Can you work these out from the model? Positions are in its coordinate system, mm. Face numbers are marked on the shaded views. A direction names the side the tool comes from. Give positions to 0.01 mm unless a question says otherwise; leave off trailing zeros. Order: outer loops, then holes, each group sorted by start corner. A loop starts at its lowest first (then second) coordinate and runs counter-clockwise, first axis right, second up. Notation, with made-up numbers: (-12, -39) - (1, -39) arc R25 ccw to (1, -5) - close; hole circle Ø5 at (-35, -29.75). An arc over 180 degrees is marked (long way). Use one line per item in the form item = value. Start each with the question number.
1) Please list where these lines run through material, in increasing order: probe 1 along Y at (x, z) = (39, 14); probe 2 along X at (y, z) = (-47, 35); probe 3 along Z at (x, y) = (90, -22).
2) Suppose I cut it at D-D, the plane y = -9.5. Write out the boundary of the cut face in (x, z), and give its area (3 significant figures).
3) Suppose I cut it at B-B, the plane y = -27. Write out the boundary of the cut face in (x, z), and give its area (3 significant figures).
4) Suppose I cut it at A-A, the plane y = -20. Write out the boundary of the cut face in (x, z), and give its area (3 significant figures).
5) Suppose I cut it at C-C, the plane x = 90. Write out the boundary of the cut face in (y, z).
6) Which directions (+Z, -Z, +X, -X, +Y, -Y) give clear straight access to the entire face, cutting with the end or side of a thin tool? Please do the marked faces 5, 6 and 7.
7) We'd pull the mould along X, two halves only. Please class the marked faces 1, 2, 3 and 4: released by +X, released by -X, zero draft, split by the parting line, or undercut.
8) For pin 1 (10 mm diameter, centred on y = -8, z = 35, fed in from -X); pin 2 (10 mm diameter, centred on x = 59, z = 23.5, fed in from +Y); pin 3 (4 mm diameter, centred on y = -21, z = 47.5, fed in from -X), each with a flat end and sliding along its axis, tell me the tip position at first contact or that it passes through.
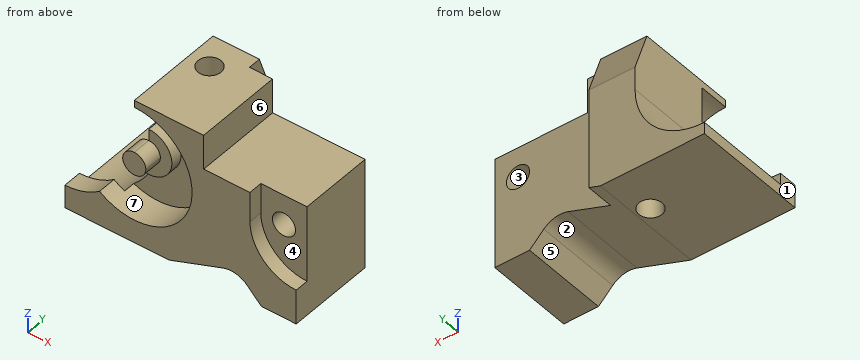
```python
from build123d import *

# Parameters (mm, degrees)
F0_W      = 100
F0_H      = 63
F1_DEPTH  = 50
F2_W      = 40
F2_H      = 15
F3_DEPTH  = 50.001
F5_DEPTH  = 6
F6_R      = 5
F7_DEPTH  = 44.001
F8_R      = 25
F9_DEPTH  = 13
F10_R     = 10
F11_DEPTH = 5
F13_DEPTH = 42
F15_DEPTH = 50.001
F17_DEPTH = 8
F19_DEPTH = 63.001
F20_R     = 5
F21_DEPTH = 63.001
F23_DEPTH = 70.001


with BuildPart() as f1:
    # F0 (on Front) → F1 (new body)
    with BuildSketch(Plane.XZ):
        with Locations((50, 31.5)):
            Rectangle(F0_W, F0_H)
    extrude(amount=F1_DEPTH)

    # F2 (on face) → F3 (cut, through all)
    with BuildSketch(Plane.XZ.offset(50)):
        with Locations((80, 55.5)):
            Rectangle(F2_W, F2_H)
        with BuildLine():
            Line((45, 0), (85, 0))
            Line((85, 0), (78.8309201782, 6.1690798218))
            ThreePointArc((78.8309201782, 6.1690798218), (73.9242485057, 8.8609720811), (68.3396509331, 8.4949382178))
            Line((68.3396509331, 8.4949382178), (45, 0))
        make_face()
    extrude(amount=-F3_DEPTH, mode=Mode.SUBTRACT)

    # F4 (on face) → F5 (cut)
    with BuildSketch(Plane.XZ.offset(50)):
        with BuildLine():
            Line((100, 48), (84.8013158464, 48))
            ThreePointArc((84.8013158464, 48), (81.2386876382, 41.9291527956), (80, 35))
            Line((80, 35), (100, 35))
            Line((100, 35), (100, 48))
        make_face()
        with BuildLine():
            ThreePointArc((80, 35), (81.2386876382, 41.9291527956), (84.8013158464, 48))
            Line((84.8013158464, 48), (80, 48))
            Line((80, 48), (80, 35))
        make_face()
        with BuildLine():
            ThreePointArc((80, 35), (85.8578643763, 20.8578643763), (100, 15))
            Line((100, 15), (100, 35))
            Line((100, 35), (80, 35))
        make_face()
    extrude(amount=-F5_DEPTH, mode=Mode.SUBTRACT)

    # F6 (on face) → F7 (cut, through all)
    with BuildSketch(Plane.XZ.offset(44)):
        with Locations((90, 35)):
            Circle(F6_R)
    extrude(amount=-F7_DEPTH, mode=Mode.SUBTRACT)

    # F8 (on face) → F9 (cut)
    with BuildSketch(Plane.XZ.offset(50)):
        with Locations((30, 35)):
            Circle(F8_R)
    extrude(amount=-F9_DEPTH, mode=Mode.SUBTRACT)

    # F10 (on face) → F11 (join)
    with BuildSketch(Plane.XZ.offset(37)):
        with Locations((30, 35)):
            Circle(F10_R)
    extrude(amount=F11_DEPTH)

    # F12 (on face) → F13 (cut)
    with BuildSketch(Plane(origin=(0, 0, 0), x_dir=(-1, 0, 0), z_dir=(0, 1, 0))):
        with BuildLine():
            ThreePointArc((-30, 35), (-24.7296369608, 51.9836702684), (-10.7703296143, 63))
            Line((-10.7703296143, 63), (-30, 63))
            Line((-30, 63), (-30, 35))
        make_face()
        with BuildLine():
            Line((0, 63), (-10.7703296143, 63))
            ThreePointArc((-10.7703296143, 63), (-24.7296369608, 51.9836702684), (-30, 35))
            Line((-30, 35), (0, 35))
            Line((0, 35), (0, 63))
        make_face()
        with BuildLine():
            ThreePointArc((-30, 35), (-21.2132034356, 13.7867965644), (0, 5))
            Line((0, 5), (0, 35))
            Line((0, 35), (-30, 35))
        make_face()
    extrude(amount=-F13_DEPTH, mode=Mode.SUBTRACT)

    # F14 (on face) → F15 (cut, through all)
    with BuildSketch(Plane(origin=(0, 0, 0), x_dir=(-1, 0, 0), z_dir=(0, 1, 0))):
        with BuildLine():
            ThreePointArc((0, 10), (17.6776695297, 17.3223304703), (25, 35))
            ThreePointArc((25, 35), (17.6776695297, 52.6776695297), (0, 60))
            Line((0, 60), (0, 35))
            Line((0, 35), (0, 10))
        make_face()
        with BuildLine():
            Line((0, 35), (0, 60))
            ThreePointArc((0, 60), (-17.6776695297, 52.6776695297), (-25, 35))
            Line((-25, 35), (0, 35))
        make_face()
        with BuildLine():
            ThreePointArc((-25, 35), (-17.6776695297, 52.6776695297), (0, 60))
            Line((0, 60), (0, 63))
            Line((0, 63), (-30, 63))
            Line((-30, 63), (-30, 35))
            Line((-30, 35), (-25, 35))
        make_face()
        with BuildLine():
            ThreePointArc((-25, 35), (-17.6776695297, 17.3223304703), (0, 10))
            Line((0, 10), (0, 35))
            Line((0, 35), (-25, 35))
        make_face()
    extrude(amount=-F15_DEPTH, mode=Mode.SUBTRACT)

    # F16 (on face) → F17 (join, through all)
    with BuildSketch(Plane.XZ.offset(42)):
        with BuildLine():
            Line((30, 35), (30, 40))
            ThreePointArc((30, 40), (25.0043497313, 35.2085147299), (29.5833333333, 30.017391357))
            ThreePointArc((29.5833333333, 30.017391357), (29.8956518578, 32.5), (30, 35))
        make_face()
        with BuildLine():
            ThreePointArc((29.5833333333, 30.017391357), (33.3850160019, 31.320099639), (35, 35))
            ThreePointArc((35, 35), (33.5355339059, 38.5355339059), (30, 40))
            Line((30, 40), (30, 35))
            ThreePointArc((30, 35), (29.8956518578, 32.5), (29.5833333333, 30.017391357))
        make_face()
    extrude(amount=F17_DEPTH)

    # F18 (on face) → F19 (cut, through all)
    with BuildSketch(Plane.XY.offset(63)):
        Polygon((100, -12), (100, 0), (60, 0), (50, 0), (50, -12), align=None)
    extrude(amount=-F19_DEPTH, mode=Mode.SUBTRACT)

    # F20 (on face) → F21 (cut, through all)
    with BuildSketch(Plane.XY.offset(63)):
        with Locations((39, -20)):
            Circle(F20_R)
    extrude(amount=-F21_DEPTH, mode=Mode.SUBTRACT)

    # F22 (on face) → F23 (cut, through all)
    with BuildSketch(Plane(origin=(30, 0, 0), x_dir=(0, -1, 0), z_dir=(-1, 0, 0))):
        Polygon((6.5514642168, 63), (0, 63), (0, 45), align=None)
    extrude(amount=-F23_DEPTH, mode=Mode.SUBTRACT)


solid = f1.part
```
Result sheet:
q1.probe_1 = -37 to -25, -15 to 0
q1.probe_2 = 25 to 35, 55 to 80
q1.probe_3 = 0 to 30, 40 to 48
q2.outline = (0, 0) - (45, 0) - (50, 1.82) - (50, 63) - (30, 63) - (30, 35) arc R30 cw to (0, 5) - close
q2.area = 1,600 mm²
q3.outline = (0, 0) - (45, 0) - (68.34, 8.49) arc R10 cw to (78.83, 6.17) - (85, 0) - (100, 0) - (100, 48) - (60, 48) - (60, 63) - (30, 63) - (30, 35) arc R30 cw to (0, 5) - close; hole circle Ø10 at (90, 35)
q3.area = 3,870 mm²
q4.outline = (0, 0) - (34, 0) - (34, 63) - (30, 63) - (30, 35) arc R30 cw to (0, 5) - close; (44, 0) - (45, 0) - (68.34, 8.49) arc R10 cw to (78.83, 6.17) - (85, 0) - (100, 0) - (100, 48) - (60, 48) - (60, 63) - (44, 63) - close; hole circle Ø10 at (90, 35)
q4.area = 3,240 mm²
q5.outline = (-50, 0) - (-12, 0) - (-12, 30) - (-44, 30) - (-44, 17.68) - (-50, 17.68) - close; (-44, 40) - (-12, 40) - (-12, 48) - (-44, 48) - close
q6.face_5 = -Z, +Y, -Y
q6.face_6 = +Z, +X, +Y, -Y
q6.face_7 = -Y
q7.face_1 = released by -X
q7.face_2 = undercut
q7.face_3 = undercut
q7.face_4 = zero draft
q8.pin_1 = 29.58
q8.pin_2 = -12
q8.pin_3 = 30
